Build history of the part. All positions in model axes, mm. A direction names the side the tool comes from. Round coordinates to 2 decimals unless told otherwise and drop trailing zeros. Loops run counter-clockwise (first coordinate to the right, second up) from the corner with the lowest first, then second, coordinate; pieces in that order, holes last. Notation, with made-up numbers: (39, -27) -> (90, -27) arc R8 cw to (90, -21) -> close; hole circle Ø6 at (-4.5, 58.5). An arc over 180 degrees is marked (long way). Put each result on its own line as item: value. Start each with the question number.
```python
from build123d import *

# Parameters (mm, degrees)
SKETCH_1_R      = 2.75
SKETCH_1_R_2    = 2
EXTRUDE_1_DEPTH = 9
SKETCH_1_6_R    = 2.75
EXTRUDE_4_DEPTH = 1
SKETCH_1_7_W    = 12.2
SKETCH_1_7_H    = 4.7
EXTRUDE_5_DEPTH = 13.5
FILLET_1_R      = 0.2


with BuildPart() as part:
    # Sketch 1 → Extrude 1 (new body)
    with BuildSketch(Plane.XY):
        with Locations((7.5, 3.5)):
            Circle(SKETCH_1_R)
        with Locations((7.5, 3.5)):
            Circle(SKETCH_1_R_2, mode=Mode.SUBTRACT)
        with BuildLine():
            ThreePointArc((8.928285686, 5.85), (7.5, 6.25), (6.071714314, 5.85))
            Line((6.071714314, 5.85), (8.928285686, 5.85))
        make_face()
        with BuildLine():
            Line((8.928285686, 1.15), (6.071714314, 1.15))
            ThreePointArc((6.071714314, 1.15), (7.5, 0.75), (8.928285686, 1.15))
        make_face()
    extrude(amount=EXTRUDE_1_DEPTH)

    # Sketch 1_6 → Extrude 4 (add)
    with BuildSketch(Plane.XY):
        with BuildLine():
            ThreePointArc((0, 1.5), (0.439339828, 0.439339828), (1.5, 0))
            Line((1.5, 0), (13.5, 0))
            ThreePointArc((13.5, 0), (14.560660172, 0.439339828), (15, 1.5))
            Line((15, 1.5), (15, 5.5))
            ThreePointArc((15, 5.5), (14.560660172, 6.560660172), (13.5, 7))
            Line((13.5, 7), (1.5, 7))
            ThreePointArc((1.5, 7), (0.439339828, 6.560660172), (0, 5.5))
            Line((0, 5.5), (0, 1.5))
        make_face()
        with Locations((7.5, 3.5)):
            Circle(SKETCH_1_6_R, mode=Mode.SUBTRACT)
    extrude(amount=EXTRUDE_4_DEPTH)

    # Sketch 1_7 → Extrude 5 (add)
    with BuildSketch(Plane.XY):
        with BuildLine():
            ThreePointArc((0, 5.5), (0.439339828, 6.560660172), (1.5, 7))
            Line((1.5, 7), (13.5, 7))
            ThreePointArc((13.5, 7), (14.560660172, 6.560660172), (15, 5.5))
            Line((15, 5.5), (15, 1.5))
            ThreePointArc((15, 1.5), (14.560660172, 0.439339828), (13.5, 0))
            Line((13.5, 0), (1.5, 0))
            ThreePointArc((1.5, 0), (0.439339828, 0.439339828), (0, 1.5))
            Line((0, 1.5), (0, 5.5))
        make_face()
        with Locations((7.5, 3.5)):
            Rectangle(SKETCH_1_7_W, SKETCH_1_7_H, mode=Mode.SUBTRACT)
        with BuildLine():
            ThreePointArc((8.928285686, 5.85), (7.5, 6.25), (6.071714314, 5.85))
            Line((6.071714314, 5.85), (8.928285686, 5.85))
        make_face()
        with BuildLine():
            Line((8.928285686, 1.15), (6.071714314, 1.15))
            ThreePointArc((6.071714314, 1.15), (7.5, 0.75), (8.928285686, 1.15))
        make_face()
    extrude(amount=-EXTRUDE_5_DEPTH)

    # Fillet 1
    fillet_1_edges = [part.edges().sort_by_distance(p)[0] for p in [
        (0.439339828, 6.560660172, 1),
        (0, 3.5, 1),
        (0.439339828, 0.439339828, 1),
        (14.560660172, 6.560660172, 1),
        (7.5, 7, 1),
        (7.5, 0, 1),
        (14.560660172, 0.439339828, 1),
        (15, 3.5, 1),
        (15, 3.5, -13.5),
        (14.560660172, 0.439339828, -13.5),
        (7.5, 0, -13.5),
        (0.439339828, 6.560660172, -13.5),
        (7.5, 7, -13.5),
        (14.560660172, 6.560660172, -13.5),
        (0.439339828, 0.439339828, -13.5),
        (0, 3.5, -13.5),
        (9.896902755, 2.151906093, 9),
    ]]
    fillet(fillet_1_edges, radius=FILLET_1_R)


solid = part.part
```
Item 1: Cut at B-B on x = 7.5. Write the cut outline in (y, z).
Item 2: Wall check: line 1 (Y direction, x = 7.5, z = 4.25); line 2 (Y direction, x = 2, z = -3.75); line 3 (Z direction, x = 12.25, y = 0.75). Give the ranges that are in metal, low to high. Write a range as from..to.
Item 3: Pull direction X, two halves, no side cores. Call faces 3 (the face through (1.4, 3, -7)), 4 (the face through (14.55, 6.57, -6.15)), 5 (the face through (6.06, 5.1, 0)), 6 (the face through (7, 7, -6)): +X half, -X half, draft (parallel to the pull), parting line (faces both ways), or undercut.
Item 4: Cut at D-D on x = 2.5. Write the cut outline in (y, z), then the cut area to 3 significant figures.
Item 5: 3-axis set-ups, long thin cutter, end or side, ignore diameter. For faces 1 (the face through (8, 1.15, -7)), 2 (the face through (15, 4, -6)): which of +Z, -Z, +X, -X, +Y, -Y reach the whole face in a straight line?
Item 6: Cut at C-C on z = -0.5. Write the cut outline in (x, y), then the cut area to 3 significant figures.
Item 7: Drop flat-ended pins along their axis: pin 1 (1 mm diameter, centred on x = 2, y = 6, fed in from +Z); pin 2 (1.4 mm diameter, centred on x = 10.5, y = 3, fed in from -Z). Give the stop position or say it passes through.
Item 8: Cut at A-A on y = 3.5. Write the cut outline in (x, z).
Ans:
1. outline: (0, -13.3) arc R0.2 ccw to (0.2, -13.5) -> (1.15, -13.5) -> (1.15, 0) -> (1.5, 0) -> (1.5, 9) -> (0.95, 9) arc R0.2 ccw to (0.75, 8.8) -> (0.75, 1) -> (0.2, 1) arc R0.2 ccw to (0, 0.8) -> close; (5.5, 0) -> (5.85, 0) -> (5.85, -13.5) -> (6.8, -13.5) arc R0.2 ccw to (7, -13.3) -> (7, 0.8) arc R0.2 ccw to (6.8, 1) -> (6.25, 1) -> (6.25, 8.8) arc R0.2 ccw to (6.05, 9) -> (5.5, 9) -> close
2. line 1: y = 0.75..1.5, 5.5..6.25
2. line 2: y = 0..1.15, 5.85..7
2. line 3: z = -13.5..1
3. face 3: undercut
3. face 4: +X half
3. face 5: undercut
3. face 6: draft
4. outline: (0, -13.3) arc R0.2 ccw to (0.2, -13.5) -> (1.15, -13.5) -> (1.15, 0) -> (5.85, 0) -> (5.85, -13.5) -> (6.8, -13.5) arc R0.2 ccw to (7, -13.3) -> (7, 0.8) arc R0.2 ccw to (6.8, 1) -> (0.2, 1) arc R0.2 ccw to (0, 0.8) -> close
4. area: 38.0 mm2
5. face 1: -Z
5. face 2: +Z, -Z, +X, +Y, -Y
6. outline: (0, 1.5) arc R1.5 ccw to (1.5, 0) -> (13.5, 0) arc R1.5 ccw to (15, 1.5) -> (15, 5.5) arc R1.5 ccw to (13.5, 7) -> (1.5, 7) arc R1.5 ccw to (0, 5.5) -> close; hole (1.4, 1.15) -> (13.6, 1.15) -> (13.6, 5.85) -> (1.4, 5.85) -> close
6. area: 45.7 mm2
7. pin 1: stops at z = 1
7. pin 2: stops at z = 0
8. outline: (0, -13.3) arc R0.2 ccw to (0.2, -13.5) -> (1.4, -13.5) -> (1.4, 0) -> (5.5, 0) -> (5.5, 9) -> (4.95, 9) arc R0.2 ccw to (4.75, 8.8) -> (4.75, 1) -> (0.2, 1) arc R0.2 ccw to (0, 0.8) -> close; (9.5, 0) -> (13.6, 0) -> (13.6, -13.5) -> (14.8, -13.5) arc R0.2 ccw to (15, -13.3) -> (15, 0.8) arc R0.2 ccw to (14.8, 1) -> (10.25, 1) -> (10.25, 8.8) arc R0.2 ccw to (10.05, 9) -> (9.5, 9) -> close
